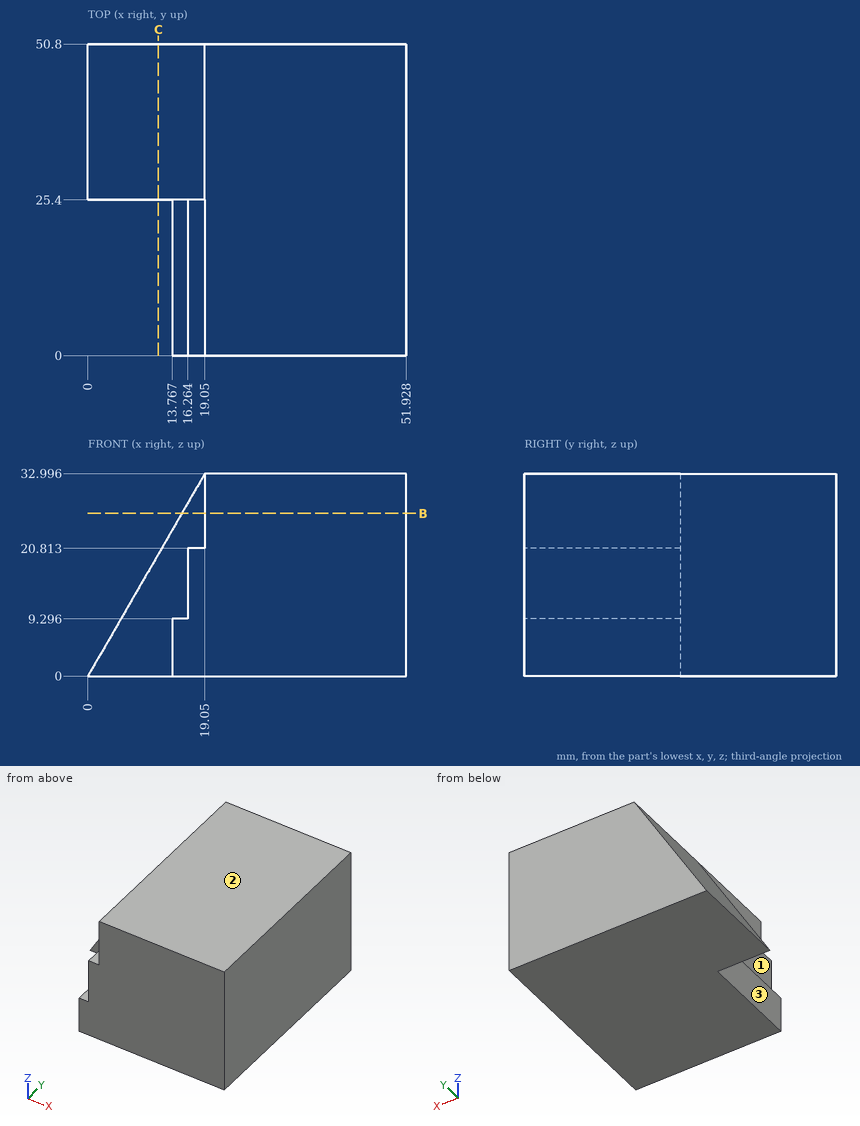
Job drawing, mm, ordinate dimensions from the low corner. One solid piece. A direction names the side the tool comes from. Give positions to 0.01 mm unless a question says otherwise; leave off trailing zeros. Loops run counter-clockwise (first coordinate to the right, second up) from the corner with the lowest first, then second, coordinate; pieces in that order, holes last. Notation, with made-up numbers: (46, 29.5) -> (104, 29.5) arc R17 ccw to (104, 58.5) -> close; hole circle Ø8 at (75.25, 88). An arc over 180 degrees is marked (long way). Write each question's results on one line, items separated by ' | '.
(1) Cut at C-C on x = 11.5. List the corners of the cut face in (y, z), and give its area (3 significant figures).
Geometry results:
outline: (25.4, 0) -> (50.8, 0) -> (50.8, 19.92) -> (25.4, 19.92) -> close | area: 506 mm²
(2) Cut at B-B on z = 26.5. List the corners of the cut face in (x, y).
Geometry results:
outline: (15.3, 25.4) -> (19.05, 25.4) -> (19.05, 0) -> (51.93, 0) -> (51.93, 50.8) -> (15.3, 50.8) -> close
(3) Probe line 1 along X through (y, z) = (3, 13.5); line 2 along Y through (x, z) = (12, 20); line 3 along X through (y, z) = (5.5, 8). List the from-to ranges inside material, lowest first.
Geometry results:
line 1: x = 16.26 to 51.93 | line 2: y = 25.4 to 50.8 | line 3: x = 13.77 to 51.93
(4) Flat gauge pins, fed straight in: pin 1 Ø1.5 at (y, z) = (31.5, 15.5) entering from -X (1 decimal); pin 2 Ø6 at (y, z) = (13.5, 29.5) entering from -X; pin 3 Ø1.2 at (x, y) = (14.5, 17.5) entering from +Z; pin 4 Ø1.5 at (x, z) = (16, 12) entering from -Y. Where does each tip first touch, or does it go through?
Geometry results:
pin 1: stops at x = 8.5 | pin 2: stops at x = 19.05 | pin 3: stops at z = 9.3 | pin 4: stops at y = 0
(5) Tool access for the marked faces 1, 2 and 3: list every direction of +Z, -Z, +X, -X, +Y, -Y with a clear straight run to the whole face (end or side of a thin tool).
Geometry results:
face 1: +Z, -X, -Y | face 2: +Z, +X, -X, +Y, -Y | face 3: +Z, -Z, -X, -Y
